from build123d import *
from build123d.topology import SkipClean

# Parameters (mm, degrees)
SKETCH_1_W           = 5.25
SKETCH_1_H           = 1.3
CUT_EXTRUDE_START    = -2.9
SKETCH_2_OUTSIDE_W   = 16.408
SKETCH_2_OUTSIDE_H   = 16.408
SKETCH_2_OUTSIDE_W_2 = 15
SKETCH_2_OUTSIDE_H_2 = 3.6
CUT_EXTRUDE_1_DEPTH  = 10
CUT_EXTRUDE_2_REACH  = 17.445
SKETCH_3_R           = 2.675


with BuildPart() as part:
    # Sketch 1 → Revolve 1 (revolve)
    with SkipClean():  # the faces are left unmerged after this step: merging them gives an invalid solid
        with BuildSketch(Plane(origin=(0, 0, 0), x_dir=(1, 0, 0), z_dir=(0, 1, 0))):
            with BuildLine():
                ThreePointArc((0, 12.7), (-4.25, 8.45), (0, 4.2))
                Line((0, 4.2), (0, 5.55))
                ThreePointArc((0, 5.55), (-2.9, 8.45), (0, 11.35))
                Line((0, 11.35), (0, 12.7))
            make_face()
            with BuildLine():
                Line((0, 5.55), (0, 4.2))
                ThreePointArc((0, 4.2), (3.00520382, 5.44479618), (4.25, 8.45))
                ThreePointArc((4.25, 8.45), (3.00520382, 11.45520382), (0, 12.7))
                Line((0, 12.7), (0, 11.35))
                ThreePointArc((0, 11.35), (2.050609665, 10.500609665), (2.9, 8.45))
                ThreePointArc((2.9, 8.45), (2.050609665, 6.399390335), (0, 5.55))
            make_face()
            with BuildLine():
                Line((0, 4.2), (0, 1.3))
                Line((0, 1.3), (4.25, 1.3))
                Line((4.25, 1.3), (4.25, 8.45))
                ThreePointArc((4.25, 8.45), (3.00520382, 5.44479618), (0, 4.2))
            make_face()
            with Locations((2.625, 0.65)):
                Rectangle(SKETCH_1_W, SKETCH_1_H)
        revolve(axis=Axis((0, 0, -1.3), (0, 0, -1)))
    add(part.part.scale(1), mode=Mode.REPLACE)  # the faces are merged on a copy

    # Sketch 2 outside → Cut-Extrude 1 (cut)
    with BuildSketch(Plane.XY.offset(CUT_EXTRUDE_START)):
        Rectangle(SKETCH_2_OUTSIDE_W, SKETCH_2_OUTSIDE_H)
        Rectangle(SKETCH_2_OUTSIDE_W_2, SKETCH_2_OUTSIDE_H_2, mode=Mode.SUBTRACT)
    extrude(amount=-CUT_EXTRUDE_1_DEPTH, mode=Mode.SUBTRACT)

    # Sketch 3 → Cut-Extrude 2 (cut, up to next)
    with BuildSketch(Plane(origin=(0, 1.8, 0), x_dir=(1, 0, 0), z_dir=(0, 1, 0)), mode=Mode.PRIVATE) as cut_extrude_2_sk1:
        with Locations(Location((0, 8.45, 0), (0, 0, 270))):
            Circle(SKETCH_3_R)
    cut_extrude_2_tool1 = extrude(cut_extrude_2_sk1.sketch, amount=-CUT_EXTRUDE_2_REACH, mode=Mode.PRIVATE) & part.part
    add(cut_extrude_2_tool1.solids().sort_by_distance((0, 1.8, -8.45))[0], mode=Mode.SUBTRACT)


solid = part.part
The model under review builds one solid part; all positions refer to its coordinate system, in mm. A direction names the side the tool comes from. Give positions to 0.01 mm unless a question says otherwise; leave off trailing zeros. Write each loop counter-clockwise with the first axis right and the second up, starting at its lowest first coordinate (ties: lowest second). Pieces come first, ordered by that corner, then holes. Notation, with made-up numbers: M 26,-33 L 77,-33 A17 ccw 77,-18 Z; hole C 68.25,24 d10. An arc over 180 degrees is marked long. One line per question, with ' | ' between items. Start each with the question number.
Item 1: We need section A-A on y = 0. Write out the cut boundary in (x, z).
Item 2: Wall thickness on line 1 (Z direction, x = -2, y = 2.5); line 2 (Z direction, x = -4.5, y = -0.5); line 3 (Y direction, x = 2.5, z = -11): over which ranges is each line inside the solid? List them lowest first. Write a range as from..to.
Item 3: We need section B-B on z = -6.5. Write out the cut boundary in (x, y).
Item 4: For faces 1 (the cylindrical face through (4.054, -1.277, -4.131)), 2 (the flat face through (0, 1.8, -5)), 3 (the cylindrical face through (-1.025, 1.465, -5.979)), 4 (the flat face through (0, -1.8, -5)), list the 3-axis set-ups (+Z, -Z, +X, -X, +Y, -Y) from which the entire face can be reached by the end or side of a thin tool; tool diameter is ignored.
Item 5: For pin 1 (3 mm diameter, centred on x = 2, z = -1.5, fed in from +Y); pin 2 (2.5 mm diameter, centred on x = -1.5, y = -3.5, fed in from -Z); pin 3 (1 mm diameter, centred on y = 4, z = -2, fed in from +X), all flat-tipped, find the tip position at first contact; note any pin that passes through.
Item 6: We need section C-C on x = -0.75. Write out the cut boundary in (y, z).
Item 7: We need section D-D on x = 3.5. Write out the cut boundary in (y, z), plus the area to 3 significant figures.
Results found:
1) outline: M -5.25,-1.3 L -4.25,-1.3 L -4.25,-8.45 A4.25 ccw 4.25,-8.45 L 4.25,-1.3 L 5.25,-1.3 L 5.25,0 L -5.25,0 Z; hole C 0,-8.45 d5.8
2) line 1: z = -2.9..0 | line 2: z = -1.3..0 | line 3: y = -1.8..1.8
3) outline: M -3.85,-1.8 L -1.17,-1.8 A2.15 cw -1.83,1.12 L -1.83,1.8 L -3.85,1.8 A4.25 ccw Z; M 1.17,-1.8 L 3.85,-1.8 A4.25 ccw 3.85,1.8 L 1.83,1.8 L 1.83,1.12 A2.15 cw Z
4) face 1: -Z | face 2: -Z, +X, -X, +Y | face 3: +Y | face 4: -Z, +X, -X, -Y
5) pin 1: stops at y = 5.22 | pin 2: stops at z = -2.9 | pin 3: stops at x = 2.41
6) outline: M -5.2,-1.3 L -4.18,-1.3 L -4.18,-2.9 L -1.8,-2.9 L -1.8,-6.3 A2.8 cw 1.12,-5.88 L 1.8,-5.88 L 1.8,-2.9 L 4.18,-2.9 L 4.18,-1.3 L 5.2,-1.3 L 5.2,0 L -5.2,0 Z; M -1.8,-12.23 A4.18 ccw 1.8,-12.23 L 1.8,-11.02 L 1.12,-11.02 A2.8 cw -1.8,-10.6 Z
7) outline: M -3.91,-1.3 L -2.41,-1.3 L -2.41,-2.9 L -1.8,-2.9 L -1.8,-10.05 A2.41 ccw 1.8,-10.05 L 1.8,-2.9 L 2.41,-2.9 L 2.41,-1.3 L 3.91,-1.3 L 3.91,0 L -3.91,0 Z | area: 45.7 mm2
